Geometry: see drawing. Coordinates: mm, zero at the bounding-box minimum. A direction names the side the tool comes from. Coordinates: 2 decimals unless noted, no trailing zeros. Write each loop counter-clockwise with the first axis right and the second up, starting at its lowest first coordinate (ties: lowest second). Pieces come first, ordered by that corner, then holes. Notation, with made-up numbers: M 74.25,60.25 L 100.25,60.25 A29 cw 100.25,90.25 Z; hole C 30.25,82 d8. An arc over 180 degrees is marked long. Answer as CSV lines item,"result". Start each with the question number.
1. Section A-A on y = 8.25. Return the cut outline in (x, z), plus the area to 4 significant figures.
2. Line query: probe 1 along X at (y, z) = (4.75, 55.5); probe 2 along Z at (x, y) = (2, 1). Output: solid intervals per line, ascending. Write a range as [from, to].
3. Section B-B on z = 42. Return the cut outline in (x, y), plus the area to 3 significant figures.
4. Contact query for flat-ended pins moving along their axis: pin 1 Ø1.5 at (y, z) = (4.5, 49) entering from -X; pin 2 Ø1 at (y, z) = (9, 37) entering from -X; pin 3 Ø2 at (x, y) = (29, 3.5) entering from +Z; pin 4 Ø3 at (y, z) = (8, 44.5) entering from +X. Output: stop coordinate, or through.
5. Reachability of the marked faces 1, 2 and 3 from +Z, -Z, +X, -X, +Y, -Y: full face, straight path, thin tool, end or side. Return the list, or none.
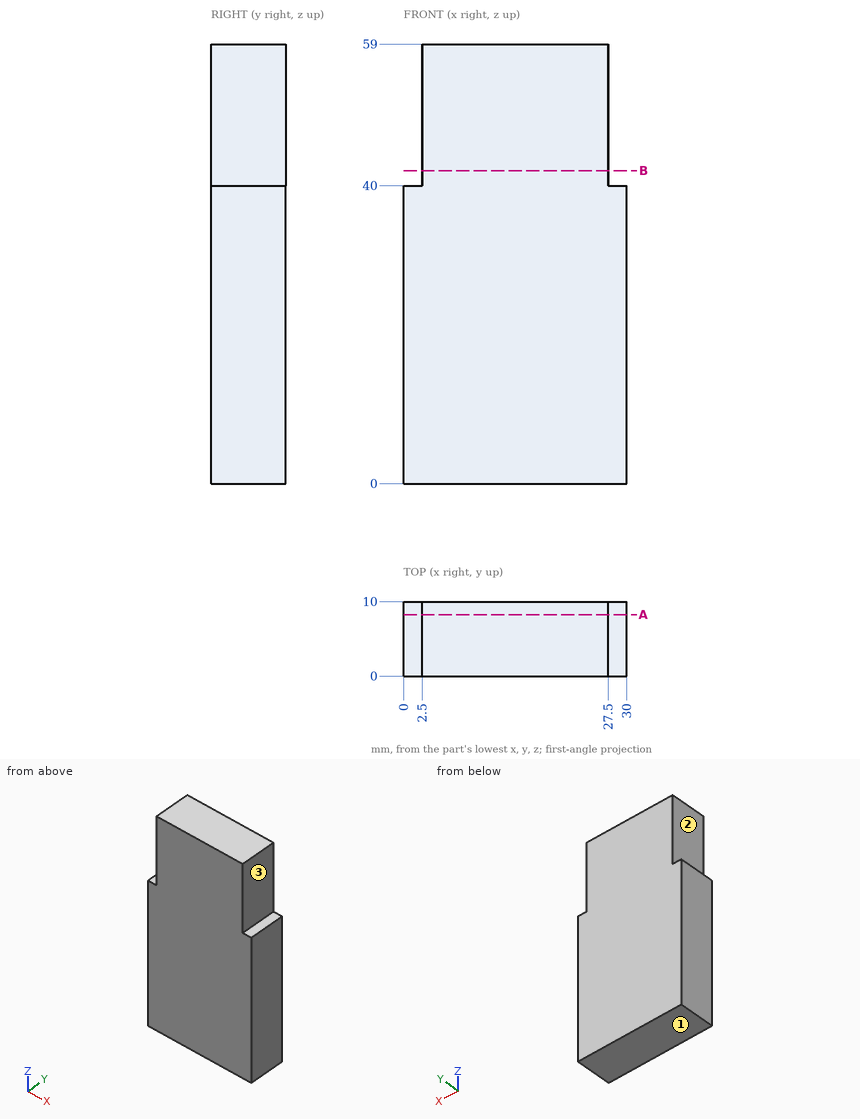
Values:
1,outline,"M 0,0 L 30,0 L 30,40 L 27.5,40 L 27.5,59 L 2.5,59 L 2.5,40 L 0,40 Z"
1,area,"1,675 mm²"
2,probe 1,"[2.5, 27.5]"
2,probe 2,"[0, 40]"
3,outline,"M 2.5,0 L 27.5,0 L 27.5,10 L 2.5,10 Z"
3,area,"250 mm²"
4,pin 1,"x = 2.5"
4,pin 2,"x = 0"
4,pin 3,"z = 40"
4,pin 4,"x = 27.5"
5,face 1,"-Z, +X, -X, +Y, -Y"
5,face 2,"+Z, -X, +Y, -Y"
5,face 3,"+Z, +X, +Y, -Y"
